Part model, mm, in its own coordinate system. A direction names the side the tool comes from. Round coordinates to 2 decimals unless told otherwise and drop trailing zeros. Write each loop counter-clockwise with the first axis right and the second up, starting at its lowest first coordinate (ties: lowest second). Pieces come first, ordered by that corner, then holes. Notation, with made-up numbers: (9, 6.5) -> (15, 6.5) arc R33 cw to (15, 40.5) -> close; hole circle Ø2 at (17, 4). An arc over 180 degrees is marked (long way). Return JSON: item names as keys, results as strings. Group by question number.
(1) Mould opens along X. For faces 4 (the flat face through (83, 3, -37)), 5 (the cylindrical face through (78.641, 5.334, -3.992)), 6 (the flat face through (0, 3, -37)) say: +X half, -X half, draft (parallel to the pull), parting line (faces both ways), or undercut.
(2) Drill centre lines: L1, parallel to X at y = 3, z = -51; L2, parallel to X at y = 5.25, z = -6; L3, parallel to Z at x = 17, y = 3.5. Where is each one in solid material? Low to high. Write a range as from..to.
(3) Drop flat-ended pins along their axis: pin 1 Ø2 at (x, y) = (74.5, 1) entering from +Z; pin 2 Ø1.6 at (x, z) = (1, -43) entering from -Y; pin 3 Ø3.5 at (x, z) = (4, -51) entering from -Y. Give the stop position or say it passes through.
(4) Saw through at B-B (y = -1.25). List the corners of the cut face in (x, z), plus the area to 3 significant figures.
(5) Saw through at A-A (z = -39). List the corners of the cut face in (x, y).
(6) Saw through at D-D (x = 18). List the corners of the cut face in (y, z), plus the area to 3 significant figures.
(7) Tool access for faces 1 (the flat face through (1, -1, -62)), 2 (the flat face through (2, 2, -37)), 3 (the cylindrical face through (4.359, 5.334, -3.992)): list every direction of +Z, -Z, +X, -X, +Y, -Y with a clear straight run to the whole face (end or side of a thin tool).
(8) Saw through at C-C (z = -66). List the corners of the cut face in (x, y), plus the area to 3 significant figures.
from build123d import *

# Parameters (mm, degrees)
BOSS_EXTRUDE1_DEPTH = 6
BOSS_EXTRUDE2_DEPTH = 1.35
SKETCH3_W           = 2
SKETCH3_H           = 10
BOSS_EXTRUDE3_DEPTH = 2.4


with BuildPart() as part:
    # Sketch1 → Boss-Extrude1 (new body)
    with BuildSketch(Plane(origin=(0, 0, 0), x_dir=(1, 0, 0), z_dir=(0, 1, 0))):
        Polygon((0, 0), (0, 72), (83, 72), (83, 0), (81, 0), (81, 70), (2, 70), (2, 0), align=None)
    extrude(amount=BOSS_EXTRUDE1_DEPTH)

    # Sketch2 → Boss-Extrude2 (add)
    with BuildSketch(Plane(origin=(0, 6, 0), x_dir=(1, 0, 0), z_dir=(0, 1, 0))):
        with BuildLine():
            Line((2, 3), (2, 70))
            Line((2, 70), (5.3, 70))
            Line((5.3, 70), (5.3, 11))
            ThreePointArc((5.3, 11), (4.8, 10.5), (5.3, 10))
            Line((5.3, 10), (5.3, 6.3))
            ThreePointArc((5.3, 6.3), (4.333452378, 3.966547622), (2, 3))
        make_face()
    boss_extrude2 = extrude(amount=-BOSS_EXTRUDE2_DEPTH)

    # Sketch3 → Boss-Extrude3 (add)
    with BuildSketch(Plane.XZ):
        with Locations((1, -5)):
            Rectangle(SKETCH3_W, SKETCH3_H)
        with Locations((1, -67)):
            Rectangle(SKETCH3_W, SKETCH3_H)
    boss_extrude3 = extrude(amount=BOSS_EXTRUDE3_DEPTH)

    # Mirror1: Boss-Extrude2, Boss-Extrude3 across plane
    add(boss_extrude2.mirror(Plane(origin=(41.5, 0, 0), x_dir=(0, 0, 1), z_dir=(1, 0, 0))))
    add(boss_extrude3.mirror(Plane(origin=(41.5, 0, 0), x_dir=(0, 0, 1), z_dir=(1, 0, 0))))


solid = part.part
Computed values:
{
 "1": {"face 4": "+X half", "face 5": "undercut", "face 6": "-X half"},
 "2": {"L1": "0..2, 81..83", "L2": "0..5.29, 77.71..83", "L3": "-72..-70"},
 "3": {"pin 1": "z = -70", "pin 2": "y = 0", "pin 3": "y = 4.65"},
 "4": {"outline": "(0, -72) -> (2, -72) -> (2, -62) -> (0, -62) -> close; (0, -10) -> (2, -10) -> (2, 0) -> (0, 0) -> close; (81, -72) -> (83, -72) -> (83, -62) -> (81, -62) -> close; (81, -10) -> (83, -10) -> (83, 0) -> (81, 0) -> close", "area": "80.0 mm2"},
 "5": {"outline": "(0, 0) -> (2, 0) -> (2, 4.65) -> (5.3, 4.65) -> (5.3, 6) -> (0, 6) -> close; (77.7, 4.65) -> (81, 4.65) -> (81, 0) -> (83, 0) -> (83, 6) -> (77.7, 6) -> close"},
 "6": {"outline": "(0, -72) -> (6, -72) -> (6, -70) -> (0, -70) -> close", "area": "12.0 mm2"},
 "7": {"face 1": "+X, -X, -Y", "face 2": "+Z, -Y", "face 3": "+Z, +Y, -Y"},
 "8": {"outline": "(0, -2.4) -> (2, -2.4) -> (2, 4.65) -> (5.3, 4.65) -> (5.3, 6) -> (0, 6) -> close; (77.7, 4.65) -> (81, 4.65) -> (81, -2.4) -> (83, -2.4) -> (83, 6) -> (77.7, 6) -> close", "area": "42.5 mm2"}
}
